Geometry: final body of the model. Coordinates: model frame, mm. Face numbers are marked on the shaded views. Round coordinates to 2 decimals unless told otherwise and drop trailing zeros. Order: outer loops, then holes, each group sorted by start corner. A loop starts at its lowest first (then second) coordinate and runs counter-clockwise, first axis right, second up. Notation, with made-up numbers: (-29.75, -18.5) -> (-6.75, -18.5) arc R30 ccw to (-6.75, 3.5) -> close; hole circle Ø8 at (66.5, 39). An arc over 180 degrees is marked (long way). Put each result on its own line as item: value.
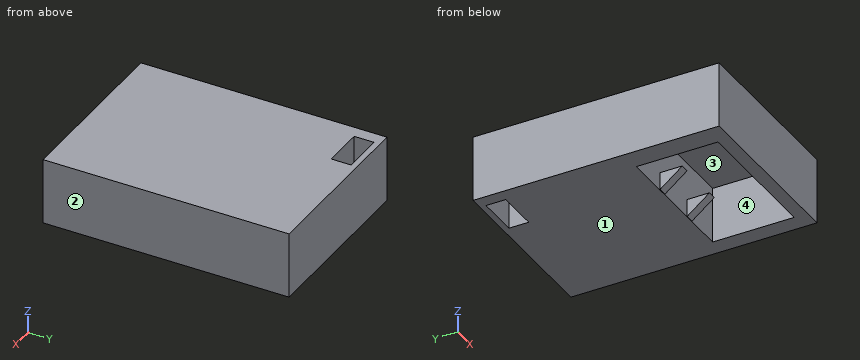
```python
from build123d import *

# Parameters (mm, degrees)
F2_DEPTH  = 25
F1_W      = 15.7
F1_H      = 7.5
F3_DEPTH  = 73
F4_W      = 52.232783
F4_H      = 30.898266
F5_DEPTH  = 21.2
F7_DEPTH  = 3.3
F10_DEPTH = 3.3


with BuildPart() as f2:
    # F0 (on Top) → F2 (new body)
    with BuildSketch(Plane.XY):
        Polygon((20.616367, 50.231609), (-46.400759, 50.231609), (-46.400759, -3.551471), (20.616367, -3.860294), align=None)
        Polygon((20.616367, -3.860294), (-46.400759, -3.551471), (-46.400759, -42.905014), (20.616367, -42.905014), align=None)
    extrude(amount=F2_DEPTH)

    # F1 (on Top) → F3 (cut)
    with BuildSketch(Plane.XY):
        with Locations((-33.749492, 44.219783)):
            Rectangle(F1_W, F1_H)
    extrude(amount=F3_DEPTH, mode=Mode.SUBTRACT)

    # F4 (on Top) → F5 (cut)
    with BuildSketch(Plane.XY):
        with Locations((-12.035032, -22.46394)):
            Rectangle(F4_W, F4_H)
    extrude(amount=F5_DEPTH, mode=Mode.SUBTRACT)

    # F6 (on Right) → F7 (join)
    with BuildSketch(Plane.YZ):
        Polygon((-15.447762, 6.884329), (-6.716418, 0), (-6.716418, 6.884329), align=None)
    extrude(amount=-F7_DEPTH)

    # F9 (on offset) → F10 (join)
    with BuildSketch(Plane.YZ.offset(-21.9)):
        Polygon((-15.447762, 6.884329), (-6.716418, 0), (-6.716418, 6.884329), align=None)
    extrude(amount=F10_DEPTH)


solid = f2.part
```
1. Cut plane C-C on z = 11.5. Return loops of the section in (x, y).
Ans:
outline: (-46.4, -42.91) -> (20.62, -42.91) -> (20.62, 50.23) -> (-46.4, 50.23) -> close; hole (-41.6, 40.47) -> (-25.9, 40.47) -> (-25.9, 47.97) -> (-41.6, 47.97) -> close; hole (-38.15, -37.91) -> (14.08, -37.91) -> (14.08, -7.01) -> (-38.15, -7.01) -> close
2. Cut plane A-A on y = 43. Return loops of the section in (x, z), and give its area (3 significant figures).
Ans:
outline: (-46.4, 0) -> (-41.6, 0) -> (-41.6, 25) -> (-46.4, 25) -> close; (-25.9, 0) -> (20.62, 0) -> (20.62, 25) -> (-25.9, 25) -> close
area: 1,280 mm²
3. Cut plane D-D on x = 6. Return loops of the section in (y, z), and give its area (3 significant figures).
Ans:
outline: (-42.91, 0) -> (-37.91, 0) -> (-37.91, 21.2) -> (-7.01, 21.2) -> (-7.01, 0) -> (50.23, 0) -> (50.23, 25) -> (-42.91, 25) -> close
area: 1,670 mm²
4. Cut plane B-B on x = -33. Return loops of the section in (y, z), and give its area (3 significant figures).
Ans:
outline: (-42.91, 0) -> (-37.91, 0) -> (-37.91, 21.2) -> (-7.01, 21.2) -> (-7.01, 0) -> (40.47, 0) -> (40.47, 25) -> (-42.91, 25) -> close; (47.97, 0) -> (50.23, 0) -> (50.23, 25) -> (47.97, 25) -> close
area: 1,490 mm²
5. Material intervals for probe 1 along Y at (x, z) = (-29, 16.5); probe 2 along Y at (x, z) = (9, 5.75); probe 3 along X at (y, z) = (44, 9), sorted ascending.
Ans:
probe 1: -42.91 to -37.91, -7.01 to 40.47, 47.97 to 50.23
probe 2: -42.91 to -37.91, -7.01 to 50.23
probe 3: -46.4 to -41.6, -25.9 to 20.62
6. Draft query along X for the marked faces 1, 2, 3 and 4. Return one class per face: +X half, -X half, draft (parallel to the pull), parting line (faces both ways), or undercut.
Ans:
face 1: draft
face 2: +X half
face 3: undercut
face 4: undercut
